```python
from build123d import *

# Parameters (mm, degrees)
F0_R          = 4.675
F0_R_2        = 3.175
F1_DEPTH      = 15
F1_DEPTH_BACK = 2.5
F2_R          = 6
F2_R_2        = 4.5
F3_DEPTH      = 15
F3_DEPTH_BACK = 2.5


# Not quite as in the source:
# - a fillet or chamfer that OpenCascade refuses, or shapes differently, is made with other operations: its cross-section is extruded or revolved along the edge and cut away or added


with BuildPart() as f1:
    # F0 (on Front) → F1 (new body, two sides)
    with BuildSketch(Plane.XZ) as f1_sk:
        Circle(F0_R)
        Circle(F0_R_2, mode=Mode.SUBTRACT)
    extrude(amount=F1_DEPTH)
    extrude(f1_sk.sketch, amount=-F1_DEPTH_BACK)

    # F2 (on Front) → F3 (join, two sides)
    with BuildSketch(Plane.XZ) as f3_sk:
        Circle(F2_R)
        Circle(F2_R_2, mode=Mode.SUBTRACT)
    extrude(amount=-F3_DEPTH)
    extrude(f3_sk.sketch, amount=F3_DEPTH_BACK)

    # F4 (on Right) → F5 (revolve)
    with BuildSketch(Plane.YZ):
        Polygon((-4.5386425355, 4.975), (-8.0257616903, 4.675), (-4.5386425355, 4.675), align=None)
        Polygon((-8.0257616903, 4.975), (-11.5128808452, 4.675), (-8.0257616903, 4.675), align=None)
        Polygon((-11.5128808452, 4.975), (-15, 4.675), (-11.5128808452, 4.675), align=None)
        Polygon((11.5128808452, 6), (15, 6), (11.5128808452, 6.3), align=None)
        Polygon((6.0257616903, 6), (9.5128808452, 6), (6.0257616903, 6.3), align=None)
        Polygon((0.5386425355, 6), (4.0257616903, 6), (0.5386425355, 6.3), align=None)
    revolve(axis=Axis((0, -13.8101289049, 0), (0, -1, 0)))

    # F6: fillet of radius 5 on 1 edges, made by hand

    # F6_s1 → F6_t2 (revolve, cut)
    with BuildSketch(Plane.XY):
        with BuildLine():
            ThreePointArc((3.175, -0.8903355291), (3.5180159975, 0.9296919432), (4.5, 2.5))
            Line((4.5, 2.5), (4.4265, 2.5678067106))
            ThreePointArc((4.4265, 2.5678067106), (3.8375, 2.6), (3.175, 2.6))
            Line((3.175, 2.6), (3.075, 2.5))
            Line((3.075, 2.5), (3.075, -0.8903355291))
            Line((3.075, -0.8903355291), (3.175, -0.8903355291))
        make_face()
    revolve(axis=Axis((0, 2.5, 0), (0, -1, 0)), mode=Mode.SUBTRACT)


solid = f1.part
```
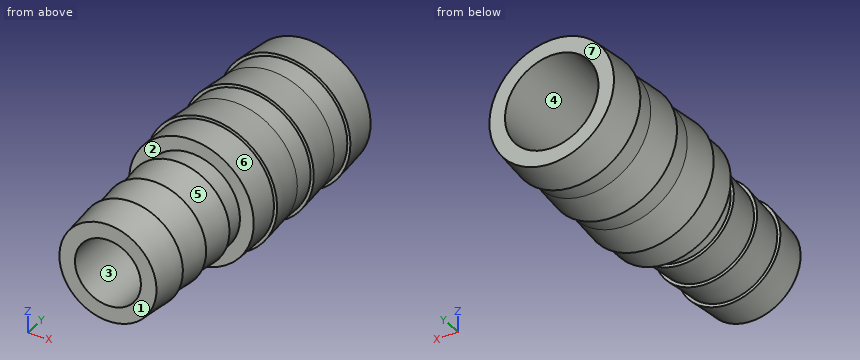
Here's how the part is built. I have some questions about the finished solid (model axes, mm). Face numbers are marked on the shaded views. A direction names the side the tool comes from. Round coordinates to 2 decimals unless told otherwise and drop trailing zeros. Loops run counter-clockwise (first coordinate to the right, second up) from the corner with the lowest first, then second, coordinate; pieces in that order, holes last. Notation, with made-up numbers: (59.25, 47) -> (81.25, 47) arc R7 ccw to (81.25, 56) -> close; hole circle Ø7 at (63, 1.5). An arc over 180 degrees is marked (long way). Answer as CSV lines item,"result". Start each with the question number.
1. For the marked faces 4, 5, 6 and 7, which set-ups out of +Z, -Z, +X, -X, +Y, -Y let a thin tool reach every point of the face, with its end or its side?
2. Imagine slicing it at A-A on y = -7.25. Write out the boundary of the cut face in (x, z) (3 decimals), plus the area to 3 significant figures.
3. Imagine slicing it at B-B on y = -12.75. Write out the boundary of the cut face in (x, z) (3 decimals), plus the area to 3 significant figures.
4. I need wall thicknesses on probe 1 along Y at (x, z) = (-5.5, -1.5); probe 2 along Z at (x, y) = (0, -5.75) (3 decimals); probe 3 along X at (y, z) = (-12, -0.75). Which ranges of each line are inside material? Lowest first, please. Write a range as from..to.
5. If we mould it in two halves opening along Y, with no side actions, what happens to the marked faces 1, 2 and 3? For each: pulls with the +Y half, pulls with the -Y half, needs draft (parallel to the pull), parting line crosses it, or undercut.
6. I'm going to push flat-ended pins straight in: P1, Ø3, axis at x = 1.5, y = 11, coming from the -Z side; P2, Ø2, axis at x = -4.5, y = 5.5, coming from the +Z side; P3, Ø3, axis at y = -2, z = -0.5, coming from the +X side. Where does each tip first touch, or does it pass through?
Solution:
1,face 4,"+Y"
1,face 5,"none"
1,face 6,"-Y"
1,face 7,"+Z, -Z, +X, -X, +Y"
2,outline,"circle Ø9.483 at (0, 0); hole circle Ø6.35 at (0, 0)"
2,area,"39.0 mm²"
3,outline,"circle Ø9.737 at (0, 0); hole circle Ø6.35 at (0, 0)"
3,area,"42.8 mm²"
4,probe 1,"-2.5..15"
4,probe 2,"-4.871..-3.175, 3.175..4.871"
4,probe 3,"-4.88..-3.09, 3.09..4.88"
5,face 1,"pulls with the -Y half"
5,face 2,"undercut"
5,face 3,"needs draft"
6,P1,"z = -6.3"
6,P2,"z = 5.14"
6,P3,"x = 6"
